```python
from build123d import *

# Parameters (mm, degrees)
CHAMFER_SIZE    = 1
CHAMFER001_SIZE = 1
SKETCH016_R     = 1.25
POCKET003_DEPTH = 3.5


with BuildPart() as part:
    # Sketch010 → Revolution (revolve)
    with BuildSketch(Plane.XZ):
        Polygon((-2.5, 9.5), (-12.5, 9.5), (-12.5, 8), (-7, 8), (-7, -11), (0, -11), (0, -4), (-2, -4), align=None)
    revolve(axis=Axis((0, 0, 0), (0, 0, 1)))

    # Chamfer
    chamfer_edges = [part.edges().sort_by_distance(p)[0] for p in [
        (2.5, 0, 9.5),
    ]]
    chamfer(chamfer_edges, length=CHAMFER_SIZE)

    # Chamfer001
    chamfer001_edges = [part.edges().sort_by_distance(p)[0] for p in [
        (7, 0, -11),
    ]]
    chamfer(chamfer001_edges, length=CHAMFER001_SIZE)

    # Sketch016 (on Face4 of Chamfer001) → Pocket003 (cut)
    with BuildSketch(Plane(origin=(0, 0, -11), x_dir=(1, 0, 0), z_dir=(0, 0, -1))):
        Circle(SKETCH016_R)
    extrude(amount=-POCKET003_DEPTH, mode=Mode.SUBTRACT)


solid = part.part
```
Geometry check sheet. Reference: the model listing, model coordinates, mm. A direction names the side the tool comes from. Round coordinates to 2 decimals unless told otherwise and drop trailing zeros. Order: outer loops, then holes, each group sorted by start corner. A loop starts at its lowest first (then second) coordinate and runs counter-clockwise, first axis right, second up. Notation, with made-up numbers: (38, 6.5) -> (71, 6.5) arc R28 ccw to (71, 40.5) -> close; hole circle Ø4 at (-15, -10). An arc over 180 degrees is marked (long way). Return JSON: item names as keys, results as strings. Group by question number.
Q1. Release check for a two-part mould opening along X. For faces 3 (the flat face through (0, 0, -7.5)), 4 (the flat face through (3, 3, 9.5)), 5 (the cylindrical face through (-6.466, 2.681, -1.126)), 6 (the flat face through (0, 0, -4)) record: released by +X, released by -X, zero draft, split by the parting line, or undercut.
Q2. Material ranges on probe 1 along Y at (x, z) = (0, -9.15); probe 2 along Z at (x, y) = (8, 1), recorded low to high. Write a range as from..to.
Q3. Gauge pin test, flat ends, axial feed: pin 1 (2 mm diameter, centred on x = 0, y = 0, fed in from -Z); pin 2 (5 mm diameter, centred on x = 3.5, z = -4, fed in from +Y); pin 3 (5 mm diameter, centred on y = 2, z = -8.5, fed in from -X). Record the tip position at first contact, or that the pin passes through.
Q4. Section check C-C, the plane z = 0. Record the boundary of the cut face in (x, y), plus the area to 3 significant figures.
Q5. Section check D-D, the plane z = -6.25. Record the boundary of the cut face in (x, y), plus the area to 3 significant figures.
Q6. Section check A-A, the plane x = 0. Record the boundary of the cut face in (y, z).
Q7. Tool access check on faces 1 (the cylindrical face through (-0.27, 1.22, -9.27)), 2 (the conical face through (0.484, 2.182, 2.338)). Record the directions out of +Z, -Z, +X, -X, +Y, -Y that give a thin tool (end or side, any length) a straight path to the whole face; none if there is none.
Numbers:
{
 "1": {"face 3": "undercut", "face 4": "zero draft", "face 5": "split by the parting line", "face 6": "undercut"},
 "2": {"probe 1": "-7..-1.25, 1.25..7", "probe 2": "8..9.5"},
 "3": {"pin 1": "z = -7.5", "pin 2": "y = 6.93", "pin 3": "x = -7"},
 "4": {"outline": "circle Ø14 at (0, 0); hole circle Ø4.3 at (0, 0)", "area": "139 mm^2"},
 "5": {"outline": "circle Ø14 at (0, 0)", "area": "154 mm^2"},
 "6": {"outline": "(-12.5, 8) -> (-7, 8) -> (-7, -10) -> (-6, -11) -> (-1.25, -11) -> (-1.25, -7.5) -> (1.25, -7.5) -> (1.25, -11) -> (6, -11) -> (7, -10) -> (7, 8) -> (12.5, 8) -> (12.5, 9.5) -> (3.5, 9.5) -> (2.46, 8.5) -> (2, -4) -> (-2, -4) -> (-2.46, 8.5) -> (-3.5, 9.5) -> (-12.5, 9.5) -> close"},
 "7": {"face 1": "-Z", "face 2": "+Z"}
}
